from build123d import *

# Parameters (mm, degrees)
BOSS_EXTRUDE1_DEPTH     = 2
SKETCH1_5_W             = 9.75
SKETCH1_5_H             = 4.75
BOSS_EXTRUDE2_DEPTH     = 12.7
CUT_EXTRUDE1_DEPTH      = 36.677198601
CUT_EXTRUDE1_DEPTH_BACK = 36.677198601
SKETCH1_6_R             = 1.7
CUT_EXTRUDE2_START      = 0.95
SKETCH2_R               = 1.2
CUT_EXTRUDE2_DEPTH      = 8


with BuildPart() as part:
    # Sketch1 → Boss-Extrude1 (new body)
    with BuildSketch(Plane(origin=(0, 0, 0), x_dir=(1, 0, 0), z_dir=(0, 1, 0))):
        Polygon((0.95, 16.25), (2.4, 16.25), (2.4, 23.65), (-5.6, 23.65), (-5.6, 16.25), (-8.8, 16.25), (-8.8, 11.5), (-17.5, 11.5), (-17.5, -8.45), (-23.5, -8.45), (-23.5, -16.45), (-17.5, -16.45), (-17.5, -16.25), (0.95, -16.25), (0.95, -16), (15.8, -16), (15.8, -8), (0.95, -8), align=None)
    extrude(amount=BOSS_EXTRUDE1_DEPTH)

    # Sketch1<5> → Boss-Extrude2 (add)
    with BuildSketch(Plane(origin=(0, 0, 0), x_dir=(1, 0, 0), z_dir=(0, 1, 0))):
        with Locations((-3.925, 13.875)):
            Rectangle(SKETCH1_5_W, SKETCH1_5_H)
        with Locations((-3.925, -13.875)):
            Rectangle(SKETCH1_5_W, SKETCH1_5_H)
    extrude(amount=-BOSS_EXTRUDE2_DEPTH)

    # Sketch1<6> → Cut-Extrude1 (cut, two sides: drawn at the far end of the back side and taken through both)
    with BuildSketch(Plane(origin=(0, 0, 0), x_dir=(1, 0, 0), z_dir=(0, 1, 0)).offset(-CUT_EXTRUDE1_DEPTH_BACK)):
        with Locations(Location((-1.6, 19.95, 0), (0, 0, 270))):
            Circle(SKETCH1_6_R)
        with Locations(Location((12.3, -12, 0), (0, 0, 270))):
            Circle(SKETCH1_6_R)
        with Locations(Location((-19.95, -12.45, 0), (0, 0, 270))):
            Circle(SKETCH1_6_R)
    extrude(amount=CUT_EXTRUDE1_DEPTH + CUT_EXTRUDE1_DEPTH_BACK, mode=Mode.SUBTRACT)

    # Sketch2 → Cut-Extrude2 (cut)
    with BuildSketch(Plane(origin=(0, 0, 0), x_dir=(0, 0, -1), z_dir=(1, 0, 0)).offset(CUT_EXTRUDE2_START)):
        with Locations(Location((-13.7, -6.45, 0), (0, 0, 180))):
            Circle(SKETCH2_R)
        with Locations(Location((13.7, -6.45, 0), (0, 0, 180))):
            Circle(SKETCH2_R)
    extrude(amount=-CUT_EXTRUDE2_DEPTH, mode=Mode.SUBTRACT)


solid = part.part
Input: part model. Units: mm. Frame: model coordinates. A direction names the side the tool comes from. Coordinates: 2 decimals unless noted, no trailing zeros. Loops run counter-clockwise (first coordinate to the right, second up) from the corner with the lowest first, then second, coordinate; pieces in that order, holes last. Notation, with made-up numbers: (-12, -27.5) -> (-5, -27.5) arc R33 cw to (-5, 10.5) -> close; hole circle Ø6 at (70.25, 52). An arc over 180 degrees is marked (long way). Write each question's results on one line, items separated by ' | '. Start each with the question number.
Q1. Pull-direction query (Y, two-part tool) for faces 1 (the flat face through (-4, 2, 1)), 2 (the flat face through (-7.05, -6, -14)), 3 (the flat face through (-5.6, 1, -20)); classes: released by +Y, released by -Y, zero draft, split by the parting line, or undercut.
Q2. Reachability of faces 4 (the flat face through (2.4, 1, -20)), 5 (the flat face through (-4, -5, 16.25)), 6 (the flat face through (-3, 0, -18)) from +Z, -Z, +X, -X, +Y, -Y: full face, straight path, thin tool, end or side. Return the list, or none.
Q3. Section B-B, the plane z = -19.95. Return the cut outline in (x, y), plus the area to 3 significant figures.
Q4. Section D-D, the plane z = 12. Return the cut outline in (x, y), plus the area to 3 significant figures.
Q5. Section A-A, the plane x = 1.5. Return the cut outline in (y, z).
Q6. Pin query (flat end, axial travel): pin 1 (4 mm diameter, centred on y = -6, z = 13, fed in from -X); pin 2 (0.7 mm diameter, centred on y = -6.5, z = -13.5, fed in from +X); pin 3 (4 mm diameter, centred on y = -5.5, z = 14, fed in from +X). Return the tip coordinate at first contact, or that it passes through.
Q7. Section C-C, the plane y = -6.45. Return the cut outline in (x, z).
Q8. Ray query, line 1 (Z direction, x = -3.5, y = -6.45); line 2 (Y direction, x = -2.25, z = 13.7); line 3 (Z direction, x = -19.95, y = 0.5). Return the intervals inside material, ascending. Write a range as from..to.
Found:
1) face 1: released by +Y | face 2: undercut | face 3: zero draft
2) face 4: -Z, +X, +Y, -Y | face 5: +Z, +X, +Y, -Y | face 6: -Z, +X, -X, -Y
3) outline: (-5.6, 0) -> (-3.3, 0) -> (-3.3, 2) -> (-5.6, 2) -> close; (0.1, 0) -> (2.4, 0) -> (2.4, 2) -> (0.1, 2) -> close | area: 9.20 mm2
4) outline: (-23.5, 0) -> (-21.59, 0) -> (-21.59, 2) -> (-23.5, 2) -> close; (-18.31, 0) -> (-8.8, 0) -> (-8.8, -12.7) -> (0.95, -12.7) -> (0.95, 0) -> (10.6, 0) -> (10.6, 2) -> (-18.31, 2) -> close; (14, 0) -> (15.8, 0) -> (15.8, 2) -> (14, 2) -> close | area: 189 mm2
5) outline: (0, -23.65) -> (2, -23.65) -> (2, -16.25) -> (0, -16.25) -> close; (0, 8) -> (2, 8) -> (2, 16) -> (0, 16) -> close
6) pin 1: x = -8.8 | pin 2: x = -7.05 | pin 3: x = 0.95
7) outline: (-8.8, -16.25) -> (0.95, -16.25) -> (0.95, -14.9) -> (-7.05, -14.9) -> (-7.05, -12.5) -> (0.95, -12.5) -> (0.95, -11.5) -> (-8.8, -11.5) -> close; (-8.8, 11.5) -> (0.95, 11.5) -> (0.95, 12.5) -> (-7.05, 12.5) -> (-7.05, 14.9) -> (0.95, 14.9) -> (0.95, 16.25) -> (-8.8, 16.25) -> close
8) line 1: -16.25..-14.9, -12.5..-11.5, 11.5..12.5, 14.9..16.25 | line 2: -12.7..-7.65, -5.25..2 | line 3: 8.45..10.75, 14.15..16.45
